Verification items for the finished model (mm, model axes). A direction names the side the tool comes from. Coordinates: 2 decimals unless noted, no trailing zeros. Order: outer loops, then holes, each group sorted by start corner. A loop starts at its lowest first (then second) coordinate and runs counter-clockwise, first axis right, second up. Notation, with made-up numbers: (1.5, 68) -> (24.5, 68) arc R27 ccw to (24.5, 95) -> close; hole circle Ø1 at (84.25, -6.75). An arc over 180 degrees is marked (long way). Write item = value, one per line. Start each with the question number.
1. Cross-section at B-B on x = 0. Record the cut outline in (y, z), plus the area to 3 significant figures.
2. Cross-section at A-A on z = 11.75. Record the cut outline in (x, y), plus the area to 3 significant figures.
3. Cross-section at D-D on y = 10.5. Record the cut outline in (x, z).
4. Thickness scan on line 1 along Y through (x, z) = (0, 0.5); line 2 along Y through (x, z) = (-13.5, 8); line 3 along X through (y, z) = (4, 9.75). Record the ranges inside material, lowest first. Write a range as from..to.
5. Release check for a two-part mould opening along Z. For faces 4 (the flat face through (4, 6, 1.4)), 5 (the cylindrical face through (4.52, 4.93, 0.71)), 6 (the cylindrical face through (-13.814, -4.75, 6.636)) record: +Z half, -Z half, draft (parallel to the pull), parting line (faces both ways), or undercut.
6. Go/stop test with flat-tipped pins: P1, Ø3, axis at y = -6, z = 8, coming from the +X side; P2, Ø7, axis at x = 0, y = 0, coming from the +Z side; P3, Ø1.3, axis at x = -6, y = 6.5, coming from the +Z side. Record where each tip stops, or that it passes through.
7. Cross-section at C-C on z = 8. Record the cut outline in (x, y).
8. Set-up check for faces 1 (the flat face through (-14, 0, 14)), 2 (the flat face through (12.8, 0, 8)), 3 (the cylindrical face through (-10.13, -0.28, 1.7)): record each of +Z, -Z, +X, -X, +Y, -Y from which the full face is reachable in a straight line by a thin tool's end or side.
from build123d import *

# Parameters (mm, degrees)
BOSS_EXTRUDE1_DEPTH = 12.7
SKETCH2_R           = 1.85
CUT_EXTRUDE1_DEPTH  = 30.6
SKETCH3_R           = 2.65
CUT_EXTRUDE2_DEPTH  = 15
SKETCH4_R           = 1.35
CUT_EXTRUDE3_DEPTH  = 3
SKETCH5_R           = 2.15
CUT_EXTRUDE4_DEPTH  = 0.6
CIRPATTERN1_COUNT   = 8
FILLET1_R           = 1


with BuildPart() as part:
    # Sketch1 → Boss-Extrude1 (new body, symmetric)
    with BuildSketch(Plane(origin=(0, 0, 0), x_dir=(1, 0, 0), z_dir=(0, 1, 0))):
        Polygon((-14.8, 0), (14.8, 0), (14.8, -14), (12.8, -14), (12.8, -2), (-12.8, -2), (-12.8, -14), (-14.8, -14), align=None)
    extrude(amount=BOSS_EXTRUDE1_DEPTH, both=True)

    # Sketch2 → Cut-Extrude1 (cut, through all)
    with BuildSketch(Plane.ZY.offset(14.8)):
        with Locations((8, -6)):
            Circle(SKETCH2_R)
        with Locations((8, 6)):
            Circle(SKETCH2_R)
    extrude(amount=-CUT_EXTRUDE1_DEPTH, mode=Mode.SUBTRACT)

    # Sketch3 → Cut-Extrude2 (cut, through all)
    with BuildSketch(Plane(origin=(0, 0, 0), x_dir=(-1, 0, 0), z_dir=(0, 0, -1))):
        Circle(SKETCH3_R)
    extrude(amount=-CUT_EXTRUDE2_DEPTH, mode=Mode.SUBTRACT)

    # Sketch4 → Cut-Extrude3 (cut, through all)
    with BuildSketch(Plane.XY.offset(2)):
        with Locations((0, 8)):
            Circle(SKETCH4_R)
    cut_extrude3 = extrude(amount=-CUT_EXTRUDE3_DEPTH, mode=Mode.SUBTRACT)

    # Sketch5 → Cut-Extrude4 (cut)
    with BuildSketch(Plane.XY.offset(2)):
        with Locations((0, 8)):
            Circle(SKETCH5_R)
    cut_extrude4 = extrude(amount=-CUT_EXTRUDE4_DEPTH, mode=Mode.SUBTRACT)

    # CirPattern1: Cut-Extrude3, Cut-Extrude4 ×8 about axis
    cirpattern1_axis = Axis((0, 0, 0), (0, 0, 1))
    for i in range(1, CIRPATTERN1_COUNT):
        add(cut_extrude3.rotate(cirpattern1_axis, i * 360 / CIRPATTERN1_COUNT), mode=Mode.SUBTRACT)
        add(cut_extrude4.rotate(cirpattern1_axis, i * 360 / CIRPATTERN1_COUNT), mode=Mode.SUBTRACT)

    # Fillet1
    fillet1_edges = [part.edges().sort_by_distance(p)[0] for p in [
        (-14.8, 0, 0),
        (14.8, 0, 0),
    ]]
    fillet(fillet1_edges, radius=FILLET1_R)


solid = part.part
Worked out:
q1.outline = (-12.7, 0) -> (-9.35, 0) -> (-9.35, 1.4) -> (-10.15, 1.4) -> (-10.15, 2) -> (-12.7, 2) -> close; (-6.65, 0) -> (-2.65, 0) -> (-2.65, 2) -> (-5.85, 2) -> (-5.85, 1.4) -> (-6.65, 1.4) -> close; (2.65, 0) -> (6.65, 0) -> (6.65, 1.4) -> (5.85, 1.4) -> (5.85, 2) -> (2.65, 2) -> close; (9.35, 0) -> (12.7, 0) -> (12.7, 2) -> (10.15, 2) -> (10.15, 1.4) -> (9.35, 1.4) -> close
q1.area = 27.5 mm²
q2.outline = (-14.8, -12.7) -> (-12.8, -12.7) -> (-12.8, 12.7) -> (-14.8, 12.7) -> close; (12.8, -12.7) -> (14.8, -12.7) -> (14.8, 12.7) -> (12.8, 12.7) -> close
q2.area = 102 mm²
q3.outline = (-14.8, 1) arc R1 ccw to (-13.8, 0) -> (13.8, 0) arc R1 ccw to (14.8, 1) -> (14.8, 14) -> (12.8, 14) -> (12.8, 2) -> (-12.8, 2) -> (-12.8, 14) -> (-14.8, 14) -> close
q4.line_1 = -12.7..-9.35, -6.65..-2.65, 2.65..6.65, 9.35..12.7
q4.line_2 = -12.7..-7.85, -4.15..4.15, 7.85..12.7
q4.line_3 = -14.8..-12.8, 12.8..14.8
q5.face_4 = +Z half
q5.face_5 = draft
q5.face_6 = undercut
q6.P1 = through
q6.P2 = 2
q6.P3 = 1.4
q7.outline = (-14.8, -12.7) -> (-12.8, -12.7) -> (-12.8, -7.85) -> (-14.8, -7.85) -> close; (-14.8, -4.15) -> (-12.8, -4.15) -> (-12.8, 4.15) -> (-14.8, 4.15) -> close; (-14.8, 7.85) -> (-12.8, 7.85) -> (-12.8, 12.7) -> (-14.8, 12.7) -> close; (12.8, -12.7) -> (14.8, -12.7) -> (14.8, -7.85) -> (12.8, -7.85) -> close; (12.8, -4.15) -> (14.8, -4.15) -> (14.8, 4.15) -> (12.8, 4.15) -> close; (12.8, 7.85) -> (14.8, 7.85) -> (14.8, 12.7) -> (12.8, 12.7) -> close
q8.face_1 = +Z, +X, -X, +Y, -Y
q8.face_2 = +Z, +Y, -Y
q8.face_3 = +Z
